Can you work these out from the model? Positions are in its coordinate system, mm. A direction names the side the tool comes from. Coordinates: 2 decimals unless noted, no trailing zeros. Order: outer loops, then holes, each group sorted by start corner. A loop starts at its lowest first (then second) coordinate and runs counter-clockwise, first axis right, second up. Notation, with made-up numbers: (-32.5, -32.75) -> (7.5, -32.75) arc R19 ccw to (7.5, -16.75) -> close; hole circle Ø3 at (41, 31.25). An arc over 180 degrees is marked (long way). Write item = value, one per line.
```python
from build123d import *

# Parameters (mm, degrees)
BOSS_EXTRUDE1_DEPTH = 12.35
SKETCH2_W           = 28.386130872
SKETCH2_H           = 32
BOSS_EXTRUDE2_DEPTH = 3


with BuildPart() as part:
    # Sketch1 → Boss-Extrude1 (new body)
    with BuildSketch(Plane.XY):
        Polygon((-155.366706922, 7.584180911), (-172.666706922, 7.584180911), (-172.666706922, 12.334180911), (-144.28057605, 12.334180911), (-144.28057605, -19.665819089), (-172.666706922, -19.665819089), (-172.666706922, -14.915819089), (-155.366706922, -14.915819089), align=None)
    extrude(amount=-BOSS_EXTRUDE1_DEPTH)

    # Sketch2 → Boss-Extrude2 (add)
    with BuildSketch(Plane.XY):
        with Locations((-158.473641486, -3.665819089)):
            Rectangle(SKETCH2_W, SKETCH2_H)
    extrude(amount=BOSS_EXTRUDE2_DEPTH)


solid = part.part
```
Item 1: I'm going to push flat-ended pins straight in: P1, Ø14, axis at x = -167.5, y = -7.5, coming from the -Z side; P2, Ø5, axis at y = -6, z = -10, coming from the -X side. Where does each tip first touch, or does it pass through?
A:
P1 = 0
P2 = -155.37
Item 2: For faces 1 (the flat face through (-164, -14.916, -6)), 2 (the flat face through (-159, -19.666, -5)), which set-ups out of +Z, -Z, +X, -X, +Y, -Y let a thin tool reach every point of the face, with its end or its side?
A:
face_1 = -Z, -X
face_2 = +Z, -Z, +X, -X, -Y
Item 3: I want a section at A-A, the plane y = -9.5. Please give me the cut outline in (x, z).
A:
outline = (-172.67, 0) -> (-155.37, 0) -> (-155.37, -12.35) -> (-144.28, -12.35) -> (-144.28, 3) -> (-172.67, 3) -> close
Item 4: I want a section at C-C, the plane z = -3.75. Please give me the cut outline in (x, y), plus the area to 3 significant figures.
A:
outline = (-172.67, -19.67) -> (-144.28, -19.67) -> (-144.28, 12.33) -> (-172.67, 12.33) -> (-172.67, 7.58) -> (-155.37, 7.58) -> (-155.37, -14.92) -> (-172.67, -14.92) -> close
area = 519 mm2
Item 5: I want a section at B-B, the plane x = -157.75. Please give me the cut outline in (y, z), plus the area to 3 significant figures.
A:
outline = (-19.67, -12.35) -> (-14.92, -12.35) -> (-14.92, 0) -> (7.58, 0) -> (7.58, -12.35) -> (12.33, -12.35) -> (12.33, 3) -> (-19.67, 3) -> close
area = 213 mm2
Item 6: If we mould it in two halves opening along Y, with no side actions, what happens to faces 3 (the flat face through (-159, 12.334, -5)), 4 (the flat face through (-144.281, -4, -5)), 5 (the flat face through (-164, -4, 0))? For each: pulls with the +Y half, pulls with the -Y half, needs draft (parallel to the pull), parting line crosses it, or undercut.
A:
face_3 = pulls with the +Y half
face_4 = needs draft
face_5 = undercut
Item 7: If I drill on probe 1 along Y at (x, z) = (-159.75, -4.5); probe 2 along X at (y, z) = (-12.5, -8); probe 3 along Z at (x, y) = (-168.75, -9), over which ranges is the centre line in solid material (lowest first)?
A:
probe_1 = -19.67 to -14.92, 7.58 to 12.33
probe_2 = -155.37 to -144.28
probe_3 = 0 to 3
